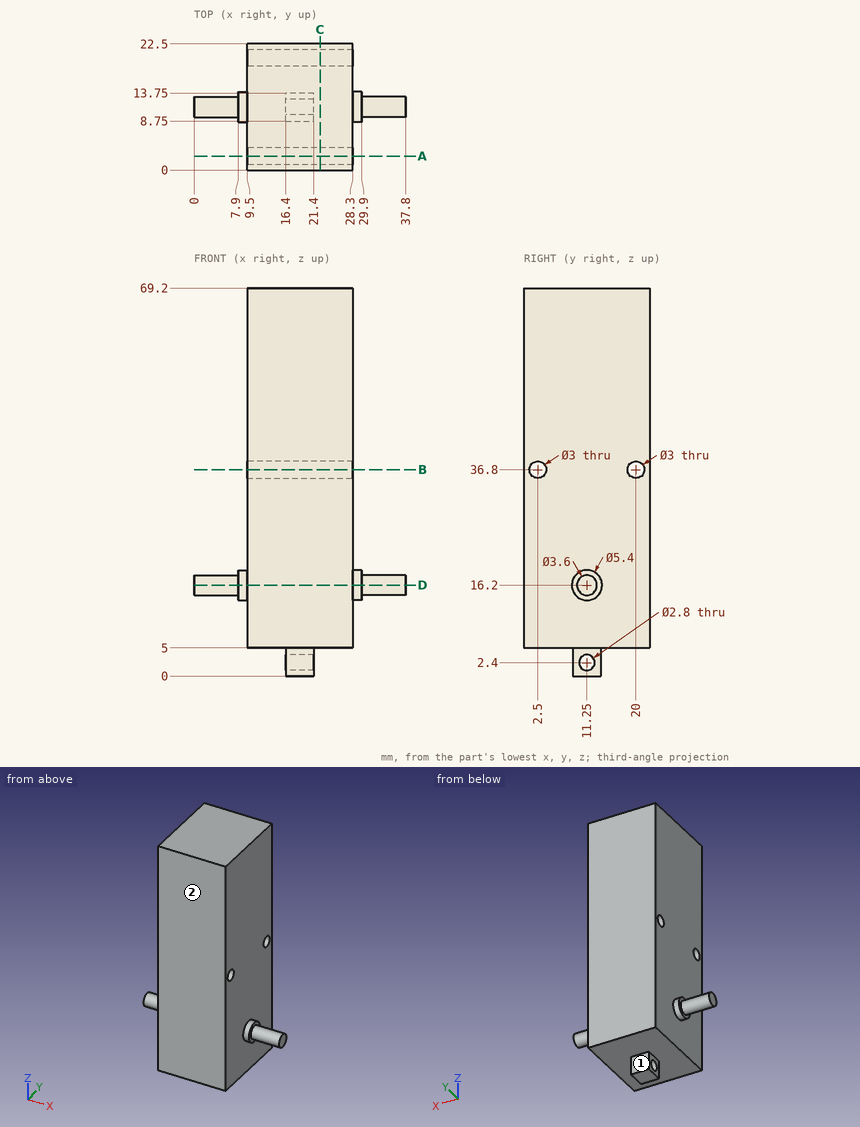
Geometry: see drawing. Coordinates: mm, zero at the bounding-box minimum. A direction names the side the tool comes from. Give positions to 0.01 mm unless a question says otherwise; leave off trailing zeros. Loops run counter-clockwise (first coordinate to the right, second up) from the corner with the lowest first, then second, coordinate; pieces in that order, holes last. Notation, with made-up numbers: (67, 0.5) -> (104, 0.5) arc R15 cw to (104, 13.5) -> close; hole circle Ø3 at (82.5, 39.25). An arc over 180 degrees is marked (long way). Use one line per item in the form item = value.
Item 1: Pin query (flat end, axial travel): P1, Ø1.5, axis at y = 12.5, z = 55.5, coming from the -X side; P2, Ø2, axis at y = 11.25, z = 2.4, coming from the +X side; P3, Ø2, axis at x = 19.5, y = 18.5, coming from the -Z side; P4, Ø3.5, axis at y = 2.5, z = 36.8, coming from the +X side. Return the tip coordinate at first contact, or that it passes through.
A:
P1 = 9.5
P2 = through
P3 = 5
P4 = 28.3
Item 2: Line query: probe 1 along Y at (x, z) = (15, 36.8); probe 2 along Y at (x, z) = (16, 36); probe 3 along Z at (x, y) = (17, 2.5). Output: solid intervals per line, ascending.
A:
probe_1 = 0 to 1, 4 to 18.5, 21.5 to 22.5
probe_2 = 0 to 1.23, 3.77 to 18.73, 21.27 to 22.5
probe_3 = 5 to 35.3, 38.3 to 69.2
Item 3: Section query D-D on z = 16.2. Output: boundary loops of the cut face in (x, y), and give its area (3 significant figures).
A:
outline = (0, 9.45) -> (7.9, 9.45) -> (7.9, 8.55) -> (9.5, 8.55) -> (9.5, 0) -> (28.3, 0) -> (28.3, 8.55) -> (29.9, 8.55) -> (29.9, 9.45) -> (37.8, 9.45) -> (37.8, 13.05) -> (29.9, 13.05) -> (29.9, 13.95) -> (28.3, 13.95) -> (28.3, 22.5) -> (9.5, 22.5) -> (9.5, 13.95) -> (7.9, 13.95) -> (7.9, 13.05) -> (0, 13.05) -> close
area = 497 mm^2
Item 4: Access query for the marked faces 1 and 2. Directions: +Z, -Z, +X, -X, +Y, -Y. A direction counts if a zero-diameter tool reaches every point of the face in a straight line with its end or side. Return the directions, or none.
A:
face_1 = -Z, +X, -X, +Y
face_2 = +Z, -Z, +X, -X, -Y
Item 5: Section query A-A on y = 2.5. Output: boundary loops of the cut face in (x, z), and give its area (3 significant figures).
A:
outline = (9.5, 5) -> (28.3, 5) -> (28.3, 35.3) -> (9.5, 35.3) -> close; (9.5, 38.3) -> (28.3, 38.3) -> (28.3, 69.2) -> (9.5, 69.2) -> close
area = 1,150 mm^2
Item 6: Section query B-B on z = 36.8. Output: boundary loops of the cut face in (x, y), and give its area (3 significant figures).
A:
outline = (9.5, 0) -> (28.3, 0) -> (28.3, 1) -> (9.5, 1) -> close; (9.5, 4) -> (28.3, 4) -> (28.3, 18.5) -> (9.5, 18.5) -> close; (9.5, 21.5) -> (28.3, 21.5) -> (28.3, 22.5) -> (9.5, 22.5) -> close
area = 310 mm^2
Item 7: Section query C-C on x = 22.5. Output: boundary loops of the cut face in (y, z), and give its area (3 significant figures).
A:
outline = (0, 5) -> (22.5, 5) -> (22.5, 69.2) -> (0, 69.2) -> close; hole circle Ø3 at (2.5, 36.8); hole circle Ø3 at (20, 36.8)
area = 1,430 mm^2
